Could you check a few things on this model? Use its own coordinates, in mm. Round coordinates to 2 decimals unless told otherwise and drop trailing zeros. Order: outer loops, then holes, each group sorted by start corner. A loop starts at its lowest first (then second) coordinate and runs counter-clockwise, first axis right, second up. Notation, with made-up numbers: (-25.75, 61.25) - (32.25, 61.25) arc R17 ccw to (32.25, 94.25) - close; hole circle Ø9 at (15, -22). An arc over 180 degrees is marked (long way). Use one line per item in the form item = value.
from build123d import *

# Parameters (mm, degrees)
SKETCH_W        = 2.5
SKETCH_H        = 2.5
PAD_DEPTH       = 2.5
CHAMFER_SIZE    = 0.3
SKETCH001_W     = 0.64
SKETCH001_H     = 0.64
PAD001_DEPTH    = 2.5
CHAMFER001_SIZE = 0.1
SKETCH002_W     = 0.64
SKETCH002_H     = 0.64
PAD002_DEPTH    = 5.5
CHAMFER002_SIZE = 0.1


with BuildPart() as part:
    # Sketch → Pad (new body)
    with BuildSketch(Plane.XY):
        with Locations((1.25, 1.25)):
            Rectangle(SKETCH_W, SKETCH_H)
    extrude(amount=PAD_DEPTH)

    # Chamfer
    chamfer_edges = [part.edges().sort_by_distance(p)[0] for p in [
        (0, 0, 1.25),
        (2.5, 0, 1.25),
        (0, 2.5, 1.25),
        (2.5, 2.5, 1.25),
    ]]
    chamfer(chamfer_edges, length=CHAMFER_SIZE)

    # Sketch001 → Pad001 (new body)
    with BuildSketch(Plane.XY.offset(2.5)):
        with Locations((1.25, 1.25)):
            Rectangle(SKETCH001_W, SKETCH001_H)
    extrude(amount=PAD001_DEPTH)

    # Chamfer001
    chamfer001_edges = [part.edges().sort_by_distance(p)[0] for p in [
        (1.25, 1.57, 5),
        (1.57, 1.25, 5),
        (1.25, 0.93, 5),
        (0.93, 1.25, 5),
    ]]
    chamfer(chamfer001_edges, length=CHAMFER001_SIZE)

    # Sketch002 → Pad002 (new body)
    with BuildSketch(Plane(origin=(0, 0, 0), x_dir=(1, 0, 0), z_dir=(0, 0, -1))):
        with Locations((1.25, -1.25)):
            Rectangle(SKETCH002_W, SKETCH002_H)
    extrude(amount=PAD002_DEPTH)

    # Chamfer002
    chamfer002_edges = [part.edges().sort_by_distance(p)[0] for p in [
        (1.25, 0.93, -5.5),
        (1.57, 1.25, -5.5),
        (1.25, 1.57, -5.5),
        (0.93, 1.25, -5.5),
    ]]
    chamfer(chamfer002_edges, length=CHAMFER002_SIZE)


solid = part.part
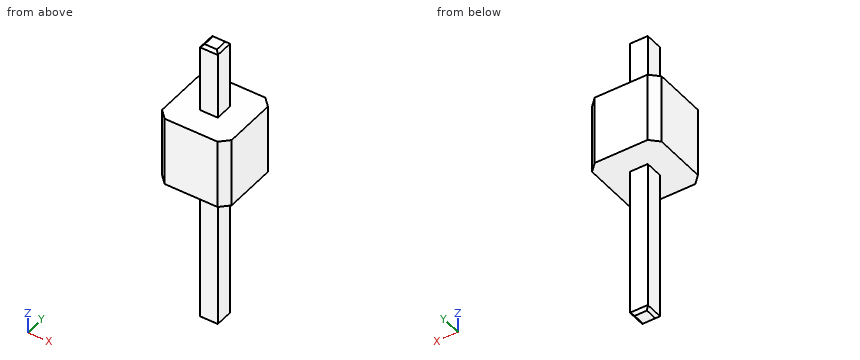
Item 1: Imagine slicing it at A-A on z = 2.25. Please give me the cut outline in (x, y), plus the area to 3 significant figures.
Found:
outline = (0, 0.3) - (0.3, 0) - (2.2, 0) - (2.5, 0.3) - (2.5, 2.2) - (2.2, 2.5) - (0.3, 2.5) - (0, 2.2) - close
area = 6.07 mm2
Item 2: I need wall thicknesses on L1, parallel to Y at x = 1.5, z = 4.25; L2, parallel to Z at x = 1.2, y = 1.85. Which ranges of each line are inside material? Lowest first, please.
Found:
L1 = 0.93 to 1.57
L2 = 0 to 2.5
Item 3: Will these pins go through, and if not, where does the flat tip stop? P1, Ø0.7, axis at x = 1, z = 3, coming from the +Y side; P2, Ø0.7, axis at y = 1, z = -3.5, coming from the -X side; P3, Ø0.5, axis at x = 1.5, z = 4, coming from the -Y side.
Found:
P1 = 1.57
P2 = 0.93
P3 = 0.93
Item 4: Imagine slicing it at B-B on x = 2.05. Please give me the cut outline in (y, z), plus the area to 3 significant figures.
Found:
outline = (0, 0) - (2.5, 0) - (2.5, 2.5) - (0, 2.5) - close
area = 6.25 mm2
